```python
from build123d import *

# Parameters (mm, degrees)
SKETCH1_R           = 17.2
SKETCH1_R_2         = 15.2
BOSS_EXTRUDE1_DEPTH = 7
SKETCH2_R           = 17.2
BOSS_EXTRUDE2_DEPTH = 2


with BuildPart() as part:
    # Sketch1 → Boss-Extrude1 (new body)
    with BuildSketch(Plane(origin=(0, 0, 0), x_dir=(1, 0, 0), z_dir=(0, 1, 0))):
        Circle(SKETCH1_R)
        Circle(SKETCH1_R_2, mode=Mode.SUBTRACT)
    extrude(amount=BOSS_EXTRUDE1_DEPTH)

    # Sketch2 → Boss-Extrude2 (add)
    with BuildSketch(Plane.XZ):
        Circle(SKETCH2_R)
        with BuildLine():
            Line((-10.9345628, 7.394277271), (-12.59131474, 8.514622313))
            ThreePointArc((-12.59131474, 8.514622313), (-8.934335835, 12.297058314), (-4.206956798, 14.606214927))
            Line((-4.206956798, 14.606214927), (-3.653409851, 12.684344542))
            ThreePointArc((-3.653409851, 12.684344542), (0, 13.2), (3.653409851, 12.684344542))
            Line((3.653409851, 12.684344542), (4.206956798, 14.606214927))
            ThreePointArc((4.206956798, 14.606214927), (8.934335835, 12.297058314), (12.59131474, 8.514622313))
            Line((12.59131474, 8.514622313), (10.9345628, 7.394277271))
            ThreePointArc((10.9345628, 7.394277271), (0, -13.2), (-10.9345628, 7.394277271))
        make_face(mode=Mode.SUBTRACT)
    extrude(amount=BOSS_EXTRUDE2_DEPTH)


solid = part.part
```
Check sheet for the modelled part. Datum: model origin and axes. Units: mm. A direction names the side the tool comes from. Round coordinates to 2 decimals unless told otherwise and drop trailing zeros. Order: outer loops, then holes, each group sorted by start corner. A loop starts at its lowest first (then second) coordinate and runs counter-clockwise, first axis right, second up. Notation, with made-up numbers: (-31, 36.25) -> (5, 36.25) arc R20 cw to (5, 62.25) -> close; hole circle Ø7 at (43, 57). An arc over 180 degrees is marked (long way). One line per item, written item: value. Start each with the question number.
Q1. Cross-section at B-B (z = -8). Record the boundary of the cut face in (x, y), and give its area (3 significant figures).
Q2. Cross-section at C-C (y = 3). Record the boundary of the cut face in (x, z), and give its area (3 significant figures).
Q3. Cross-section at D-D (x = 12). Record the boundary of the cut face in (y, z).
Q4. Cross-section at A-A (x = 0). Record the boundary of the cut face in (y, z), and give its area (3 significant figures).
Q5. Set-up check for faces 4 (the face through (3.926, -0.986, 13.632)), 5 (the face through (4, -2, -13)), 6 (the face through (-1, 0, -14)): record each of +Z, -Z, +X, -X, +Y, -Y from which the full face is reachable in a straight line by a thin tool's end or side.
Q6. Mould release check, pull along X, two halves, no side actions. Record for faces 1 (the face through (-11.751, -0.986, 7.947)), 2 (the face through (9, 7, 13)), 3 (the face through (-17.183, 2.563, 0.756)): pulls with the +X half, pulls with the -X half, needs draft (parallel to the pull), parting line crosses it, or undercut.
Q7. Thickness scan on line 1 (Z direction, x = 0, y = -0.5); line 2 (Z direction, x = 11.5, y = -1); line 3 (Z direction, x = 12, y = -1). Record the ranges inside material, lowest first.
Q8. Gauge pin test, flat ends, axial feed: pin 1 Ø1.5 at (x, y) = (-6, 1) entering from +Z; pin 2 Ø2 at (x, z) = (-1, 14) entering from +Y; pin 3 Ø4 at (y, z) = (3.5, 9) entering from +X. Record the tip position at first contact, or that the pin passes through.
Completed:
1. outline: (-15.23, -2) -> (-10.5, -2) -> (-10.5, 0) -> (-12.92, 0) -> (-12.92, 7) -> (-15.23, 7) -> close; (10.5, -2) -> (15.23, -2) -> (15.23, 7) -> (12.92, 7) -> (12.92, 0) -> (10.5, 0) -> close
1. area: 51.1 mm²
2. outline: circle Ø34.4 at (0, 0); hole circle Ø30.4 at (0, 0)
2. area: 204 mm²
3. outline: (-2, -12.32) -> (7, -12.32) -> (7, -9.33) -> (0, -9.33) -> (0, -5.5) -> (-2, -5.5) -> close; (-2, 5.5) -> (0, 5.5) -> (0, 8.11) -> (-2, 8.11) -> close; (-2, 9.33) -> (7, 9.33) -> (7, 12.32) -> (-2, 12.32) -> close
4. outline: (-2, -17.2) -> (7, -17.2) -> (7, -15.2) -> (0, -15.2) -> (0, -13.2) -> (-2, -13.2) -> close; (-2, 13.2) -> (0, 13.2) -> (0, 15.2) -> (7, 15.2) -> (7, 17.2) -> (-2, 17.2) -> close
4. area: 44.0 mm²
5. face 4: +Y, -Y
5. face 5: +Z, -Z, +X, -X, -Y
5. face 6: +Y
6. face 1: undercut
6. face 2: needs draft
6. face 3: parting line crosses it
7. line 1: z = -17.2 to -13.2, 13.2 to 17.2
7. line 2: z = -12.79 to -6.48, 6.48 to 7.78, 9.94 to 12.79
7. line 3: z = -12.32 to -5.5, 5.5 to 8.11, 9.33 to 12.32
8. pin 1: stops at z = 16.38
8. pin 2: stops at y = 0
8. pin 3: stops at x = 15.71
